```python
from build123d import *

# Parameters (mm, degrees)
F0_W     = 88
F0_H     = 30
F0_R     = 11.1
F1_DEPTH = 7
F2_SIZE  = 7.5
F3_SIZE  = 2.5


with BuildPart() as f1:
    # F0 (on Top) → F1 (new body)
    with BuildSketch(Plane.XY):
        Rectangle(F0_W, F0_H)
        with Locations((-27.5, 0)):
            Circle(F0_R, mode=Mode.SUBTRACT)
        Circle(F0_R, mode=Mode.SUBTRACT)
        with Locations((27.5, 0)):
            Circle(F0_R, mode=Mode.SUBTRACT)
    extrude(amount=F1_DEPTH)

    # F2
    f2_edges = [f1.edges().sort_by_distance(p)[0] for p in [
        (-44, -15, 3.5),
        (-44, 15, 3.5),
        (44, 15, 3.5),
        (44, -15, 3.5),
    ]]
    chamfer(f2_edges, length=F2_SIZE)

    # F3
    f3_edges = [f1.edges().sort_by_distance(p)[0] for p in [
        (0, 15, 7),
        (-40.25, 11.25, 7),
        (-44, 0, 7),
        (-40.25, -11.25, 7),
        (0, -15, 7),
        (40.25, -11.25, 7),
        (44, 0, 7),
        (40.25, 11.25, 7),
        (0, 15, 0),
        (-40.25, 11.25, 0),
        (-44, 0, 0),
        (-40.25, -11.25, 0),
        (0, -15, 0),
        (40.25, -11.25, 0),
        (44, 0, 0),
        (40.25, 11.25, 0),
    ]]
    chamfer(f3_edges, length=F3_SIZE)


solid = f1.part
```
Input: part model. Units: mm. Frame: model coordinates. Round coordinates to 2 decimals unless told otherwise and drop trailing zeros. Loops run counter-clockwise (first coordinate to the right, second up) from the corner with the lowest first, then second, coordinate; pieces in that order, holes last. Notation, with made-up numbers: (-2.75, -21.75) -> (2.25, -21.75) arc R7 cw to (2.25, -16.75) -> close; hole circle Ø9 at (-27, 27.25). An arc over 180 degrees is marked (long way). One line per item, written item: value.
(1) Pin query (flat end, axial travel): pin 1 (18 mm diameter, centred on x = -27.5, y = 0, fed in from +Z). Return the tip coordinate at first contact, or that it passes through.
Geometry check:
pin 1: through
(2) Section A-A (x = 27.5). Return the cut outline in (y, z).
Geometry check:
outline: (-15, 2.5) -> (-12.5, 0) -> (-11.1, 0) -> (-11.1, 7) -> (-12.5, 7) -> (-15, 4.5) -> close; (11.1, 0) -> (12.5, 0) -> (15, 2.5) -> (15, 4.5) -> (12.5, 7) -> (11.1, 7) -> close
(3) Section C-C (z = 3.5). Return the cut outline in (x, y), plus the area to 3 significant figures.
Geometry check:
outline: (-44, -7.5) -> (-36.5, -15) -> (36.5, -15) -> (44, -7.5) -> (44, 7.5) -> (36.5, 15) -> (-36.5, 15) -> (-44, 7.5) -> close; hole circle Ø22.2 at (-27.5, 0); hole circle Ø22.2 at (0, 0); hole circle Ø22.2 at (27.5, 0)
area: 1,370 mm2
(4) Mould query, pull axis Y, two halves, no side actions, for faces 1 (the face through (44, 0, 3)), 2 (the face through (40.3, -11.2, 3.5)), 3 (the face through (-16.9, 3.3, 3.5)). Classes: pulls with the +Y half, pulls with the -Y half, needs draft (parallel to the pull), parting line crosses it, or undercut.
Geometry check:
face 1: needs draft
face 2: pulls with the -Y half
face 3: undercut
(5) Material intervals for line 1 (X direction, y = 9, z = 5.5); line 2 (Y direction, x = -27.5, z = 3.75); line 3 (X direction, y = 1.25, z = 4.5), sorted ascending. Write a range as [from, to].
Geometry check:
line 1: [-41.09, -34], [-21, -6.5], [6.5, 21], [34, 41.09]
line 2: [-15, -11.1], [11.1, 15]
line 3: [-44, -38.53], [-16.47, -11.03], [11.03, 16.47], [38.53, 44]
(6) Section D-D (y = 4.5). Return the cut outline in (x, z), plus the area to 3 significant figures.
Geometry check:
outline: (-44, 2.5) -> (-41.5, 0) -> (-37.65, 0) -> (-37.65, 7) -> (-41.5, 7) -> (-44, 4.5) -> close; (-17.35, 0) -> (-10.15, 0) -> (-10.15, 7) -> (-17.35, 7) -> close; (10.15, 0) -> (17.35, 0) -> (17.35, 7) -> (10.15, 7) -> close; (37.65, 0) -> (41.5, 0) -> (44, 2.5) -> (44, 4.5) -> (41.5, 7) -> (37.65, 7) -> close
area: 177 mm2
(7) Section B-B (y = 0). Return the cut outline in (x, z), plus the area to 3 significant figures.
Geometry check:
outline: (-44, 2.5) -> (-41.5, 0) -> (-38.6, 0) -> (-38.6, 7) -> (-41.5, 7) -> (-44, 4.5) -> close; (-16.4, 0) -> (-11.1, 0) -> (-11.1, 7) -> (-16.4, 7) -> close; (11.1, 0) -> (16.4, 0) -> (16.4, 7) -> (11.1, 7) -> close; (38.6, 0) -> (41.5, 0) -> (44, 2.5) -> (44, 4.5) -> (41.5, 7) -> (38.6, 7) -> close
area: 137 mm2
